```python
from build123d import *

# Parameters (mm, degrees)
F0_W      = 127
F0_H      = 215.9
F1_DEPTH  = 107.95
F3_W      = 76.2
F3_H      = 44.45
F3_W_2    = 50.8
F4_DEPTH  = 76.2
F5_D      = 25.4
F7_DEPTH  = 127.001
F9_D      = 25.4
F3_H_2    = 63.5
F10_DEPTH = 50.8


with BuildPart() as f1:
    # F0 (on Top) → F1 (new body)
    with BuildSketch(Plane.XY):
        with Locations((63.5, 108.900839)):
            Rectangle(F0_W, F0_H)
    extrude(amount=F1_DEPTH)

    # F3 (on face) → F4 (cut)
    with BuildSketch(Plane.XZ.offset(-0.950839)):
        with Locations((88.9, 22.225)):
            Rectangle(F3_W, F3_H)
        with Locations((25.4, 22.225)):
            Rectangle(F3_W_2, F3_H)
    extrude(amount=-F4_DEPTH, mode=Mode.SUBTRACT)

    # F5 (through all)
    with Locations(Plane.YZ.offset(127)):
        with Locations((146.548077, 44.45)):
            Hole(F5_D / 2)

    # F6 (on face) → F7 (cut, through all)
    with BuildSketch(Plane.YZ.offset(127)):
        with BuildLine():
            ThreePointArc((150.082376, 107.95), (198.809879, 63.46501), (216.850839, 0))
            Line((216.850839, 0), (216.850839, 107.95))
            Line((216.850839, 107.95), (150.082376, 107.95))
        make_face()
    extrude(amount=-F7_DEPTH, mode=Mode.SUBTRACT)

    # F9 (through all)
    with Locations(Plane.XZ.offset(-0.950839)):
        with Locations((88.9, 76.2)):
            Hole(F9_D / 2)

    # F3 (on face) → F10 (cut)
    with BuildSketch(Plane.XZ.offset(-0.950839)):
        with Locations((25.4, 76.2)):
            Rectangle(F3_W_2, F3_H_2)
    extrude(amount=-F10_DEPTH, mode=Mode.SUBTRACT)


solid = f1.part
```
CAD build for the part. Positions are in the model's coordinates, mm. A direction names the side the tool comes from. Coordinates: 2 decimals unless noted, no trailing zeros. Order: outer loops, then holes, each group sorted by start corner. A loop starts at its lowest first (then second) coordinate and runs counter-clockwise, first axis right, second up. Notation, with made-up numbers: (68.5, 54.25) - (116.5, 54.25) arc R27 ccw to (116.5, 91.25) - close; hole circle Ø9 at (-10, 53). An arc over 180 degrees is marked (long way). Use a Markdown table: item, result. Add a question column.
(1) Saw through at C-C (x = 88.9). Give the cut face in (y, z).
(2) Flat gauge pins, fed straight in: pin 1 (15 mm diameter, centred on y = 37.5, z = 73, fed in from -X); pin 2 (12 mm diameter, centred on x = 31.5, z = 13, fed in from -Y); pin 3 (12 mm diameter, centred on x = 104, z = 70, fed in from +Y). Where does each tip first touch, or does it go through?
(3) Saw through at B-B (y = 95.5). Give the cut face in (x, z), then the cut area to 3 significant figures.
(4) Pull direction Y, two halves, no side cores. Call faces 1 (the face through (62.611, 134.817, 39.586)), 2 (the face through (64.389, 198.315, 64.259)), 3 (the face through (91.65, 101.25, 63.8)): +Y half, -Y half, draft (parallel to the pull), parting line (faces both ways), or undercut.
(5) Saw through at A-A (x = 74). Give the cut face in (y, z).
(6) Which spindle directions (+Z, -Z, +X, -X, +Y, -Y) get a long thin tool onto all of the face, cutting with end or side? Do faces 4 (the face through (79, 47, 44.45)), 5 (the face through (88, 0.951, 62)), 6 (the face through (50.8, 26, 76)). Say none if no direction does.
(7) Drill centre lines: line 1 along Z through (x, y) = (80.5, 139); line 2 along Z through (x, y) = (88.9, 66); line 3 along Z through (x, y) = (88, 136). Where is each one in solid material? Low to high. Write a range as [from, to].
(8) Saw through at D-D (z = 40.5). Give the cut face in (x, y).
Solved:
| question | item | result |
|---|---|---|
| 1 | outline | (0.95, 44.45) - (77.15, 44.45) - (77.15, 0) - (216.85, 0) arc R120.65 ccw to (198.79, 63.5) - (0.95, 63.5) - close; (0.95, 88.9) - (177.77, 88.9) arc R120.65 ccw to (150.08, 107.95) - (0.95, 107.95) - close; hole circle Ø25.4 at (146.55, 44.45) |
| 2 | pin 1 | stops at x = 50.8 |
| 2 | pin 2 | stops at y = 77.15 |
| 2 | pin 3 | stops at y = 198.48 |
| 3 | outline | (0, 0) - (127, 0) - (127, 107.95) - (0, 107.95) - close; hole circle Ø25.4 at (88.9, 76.2) |
| 3 | area | 13,200 mm² |
| 4 | face 1 | undercut |
| 4 | face 2 | +Y half |
| 4 | face 3 | draft |
| 5 | outline | (0.95, 44.45) - (77.15, 44.45) - (77.15, 0) - (216.85, 0) arc R120.65 ccw to (150.08, 107.95) - (0.95, 107.95) - close; hole circle Ø25.4 at (146.55, 44.45) |
| 6 | face 4 | -Z, +X, -X, -Y |
| 6 | face 5 | +Z, -Z, +X, -X, -Y |
| 6 | face 6 | +Z, -Z, -X, -Y |
| 7 | line 1 | z = [0, 34.24], [54.66, 66.67], [85.73, 107.95] |
| 7 | line 2 | z = [44.45, 63.5], [88.9, 107.95] |
| 7 | line 3 | z = [0, 37.38], [51.52, 63.53], [88.87, 107.95] |
| 8 | outline | (0, 77.15) - (127, 77.15) - (127, 134.48) - (0, 134.48) - close; (0, 158.62) - (127, 158.62) - (127, 209.85) - (0, 209.85) - close |
